from build123d import *

# Parameters (mm, degrees)
BOSS_EXTRUDE1_DEPTH      = 30
SKETCH3_R                = 4
CUT_EXTRUDE1_DEPTH       = 40
SKETCH4_W                = 3
SKETCH4_H                = 41
BOSS_EXTRUDE2_DEPTH      = 4
BOSS_EXTRUDE3_DEPTH      = 30
BOSS_EXTRUDE3_DEPTH_BACK = 4
SKETCH5_W                = 3
SKETCH5_H                = 7.75


with BuildPart() as part:
    # Sketch1 → Boss-Extrude1 (new body)
    with BuildSketch(Plane(origin=(0, 0, 0), x_dir=(1, 0, 0), z_dir=(0, 1, 0))):
        Polygon((-12.8, -12.8), (-13.1, 12.8), (13.1, 12.8), (12.8, -12.6), (16.799721029, -12.6472408), (17.147523085, 16.8), (-17.147149649, 16.8), (-16.79972537, -12.846871782), align=None)
    extrude(amount=BOSS_EXTRUDE1_DEPTH)

    # Sketch3 → Cut-Extrude1 (cut)
    with BuildSketch(Plane(origin=(16.946733814, 0, 0.200158273), x_dir=(0.011810199887684227, 0, -0.9999302571572745), z_dir=(0.9999302571572745, 0, 0.011810199887684227))):
        with Locations(Location((0.252049318, 15, 0), (0, 0, 180))):
            Circle(SKETCH3_R)
    extrude(amount=-CUT_EXTRUDE1_DEPTH, mode=Mode.SUBTRACT)

    # Sketch4 → Boss-Extrude2 (add)
    with BuildSketch(Plane(origin=(0, 0, -16.8), x_dir=(-1, 0, 0), z_dir=(0, 0, -1))):
        with Locations((12.499813282, 15)):
            Rectangle(SKETCH4_W, SKETCH4_H)
    extrude(amount=-BOSS_EXTRUDE2_DEPTH)

    # Sketch5 → Boss-Extrude3 (add, two sides: drawn at the far end of the back side and taken through both)
    with BuildSketch(Plane(origin=(0, 0, -16.8), x_dir=(-1, 0, 0), z_dir=(0, 0, -1)).offset(-BOSS_EXTRUDE3_DEPTH_BACK)):
        with Locations((12.499813282, 39.375)):
            Rectangle(SKETCH5_W, SKETCH5_H)
        with Locations((12.499813282, -9.375)):
            Rectangle(SKETCH5_W, SKETCH5_H)
    extrude(amount=BOSS_EXTRUDE3_DEPTH + BOSS_EXTRUDE3_DEPTH_BACK)


solid = part.part
Geometry: final body of the model. Coordinates: model frame, mm. A direction names the side the tool comes from. Coordinates: 2 decimals unless noted, no trailing zeros. Order: outer loops, then holes, each group sorted by start corner. A loop starts at its lowest first (then second) coordinate and runs counter-clockwise, first axis right, second up.
(1) Section query B-B (y = 24). Return the cut outline in (x, z).
(2) Material intervals for probe 1 along X at (y, z) = (-4.5, -14.5); probe 2 along Z at (x, y) = (-11.5, 22); probe 3 along X at (y, z) = (5, 7.5), sorted ascending.
(3) First-contact query: pin 1 (6.5 mm diameter, centred on y = -8, z = -31, fed in from -X); pin 2 (14 mm diameter, centred on x = 9.5, z = -4.5, fed in from +Y); pin 3 (5 mm diameter, centred on x = -14.5, z = -5, fed in from -Y). Flat tips, straight axial feed; report the tip coordinate or a pass-through.
(4) Section query C-C (x = -12). Return the cut outline in (y, z).
(5) Draft query along Z for faces 1 (the face through (-12, 39, -46.8)), 2 (the face through (-14.924, 11.034, -0.949)), 3 (the face through (9, 0, -13)). Return one class per face: pulls with the +Z half, pulls with the -Z half, needs draft (parallel to the pull), parting line crosses it, or undercut.
(6) Access query for faces 4 (the face through (-14, 39, -30)), 5 (the face through (0, 15, -16.8)), 6 (the face through (-11, 39, -30)). Directions: +Z, -Z, +X, -X, +Y, -Y. A direction counts if a zero-diameter tool reaches every point of the face in a straight line with its end or side. Return the directions, or none.
(7) Section query A-A (z = -37). Return the cut outline in (x, y), plus the area to 3 significant figures.
(8) Section query D-D (y = -4). Return the cut outline in (x, z), plus the area to 3 significant figures.
Solution:
1. outline: (-17.15, -16.8) - (17.15, -16.8) - (16.8, 12.65) - (12.8, 12.6) - (13.1, -12.8) - (-13.1, -12.8) - (-12.8, 12.8) - (-16.8, 12.85) - close
2. probe 1: x = -14 to -11
2. probe 2: z = -16.8 to -12.8
2. probe 3: x = -16.86 to -12.86, 12.86 to 16.86
3. pin 1: stops at x = -14
3. pin 2: stops at y = 30
3. pin 3: stops at y = 0
4. outline: (-13.25, -46.8) - (-5.5, -46.8) - (-5.5, -16.8) - (35.5, -16.8) - (35.5, -46.8) - (43.25, -46.8) - (43.25, -12.8) - (-13.25, -12.8) - close
5. face 1: pulls with the -Z half
5. face 2: undercut
5. face 3: needs draft
6. face 4: +Z, -Z, -X, +Y
6. face 5: -Z, +X, -X
6. face 6: +Z, -Z, +X, +Y
7. outline: (-14, -13.25) - (-11, -13.25) - (-11, -5.5) - (-14, -5.5) - close; (-14, 35.5) - (-11, 35.5) - (-11, 43.25) - (-14, 43.25) - close
7. area: 46.5 mm2
8. outline: (-14, -16.8) - (-11, -16.8) - (-11, -12.8) - (-14, -12.8) - close
8. area: 12.0 mm2
